Geometry: final body of the model. Coordinates: model frame, mm. Face numbers are marked on the shaded views. Give positions to 0.01 mm unless a question says otherwise; leave off trailing zeros. Order: outer loops, then holes, each group sorted by start corner. A loop starts at its lowest first (then second) coordinate and runs counter-clockwise, first axis right, second up. Notation, with made-up numbers: (3, -6) - (10, -6) arc R25 ccw to (10, 27) - close; hole circle Ø8 at (2, -12.5). An arc over 180 degrees is marked (long way). One line per item, written item: value.
```python
from build123d import *

# Parameters (mm, degrees)
MINUS_PLATE_10_X_8_5_X_0_5_SKETCH_W = 10
MINUS_PLATE_10_X_8_5_X_0_5_SKETCH_H = 0.5
MINUS_PLATE_10_X_8_5_X_0_5_DEPTH    = 8.5
SOLDER_TAB_1_5_X_2_5_SKETCH_W       = 1.5
SOLDER_TAB_1_5_X_2_5_SKETCH_H       = 0.5
SOLDER_TAB_1_5_X_2_5_DEPTH          = 2.5


with BuildPart() as part:
    # Minus Plate 10 x 8.5 x 0.5 Sketch → Minus Plate 10 x 8.5 x 0.5 (new body)
    with BuildSketch(Plane(origin=(0, 1.95, 0), x_dir=(1, 0, 0), z_dir=(0, 1, 0))):
        with Locations((25.7, 65.1)):
            Rectangle(MINUS_PLATE_10_X_8_5_X_0_5_SKETCH_W, MINUS_PLATE_10_X_8_5_X_0_5_SKETCH_H)
    extrude(amount=MINUS_PLATE_10_X_8_5_X_0_5_DEPTH)

    # Solder Tab 1.5 x 2.5 Sketch → Solder Tab 1.5 x 2.5 (add)
    with BuildSketch(Plane(origin=(0, 10.45, 0), x_dir=(1, 0, 0), z_dir=(0, 1, 0))):
        with Locations((25.7, 65.1)):
            Rectangle(SOLDER_TAB_1_5_X_2_5_SKETCH_W, SOLDER_TAB_1_5_X_2_5_SKETCH_H)
    extrude(amount=SOLDER_TAB_1_5_X_2_5_DEPTH)

    # Spring (compressed 4.3) Sketch → Spring (compressed 4.3) (revolve)
    with BuildSketch(Plane(origin=(0, 6.95, 0), x_dir=(1, 0, 0), z_dir=(0, 1, 0)), mode=Mode.PRIVATE) as spring_compressed_4_3_sk:
        Polygon((28.2, 64.85), (28.7, 64.85), (27.7, 60.55), (27.2, 60.55), align=None)
    revolve(spring_compressed_4_3_sk.sketch.rotate(Axis((25.7, 6.95, -65.85), (0, 0, 1)), 180), axis=Axis((25.7, 6.95, -65.85), (0, 0, 1)))


solid = part.part
```
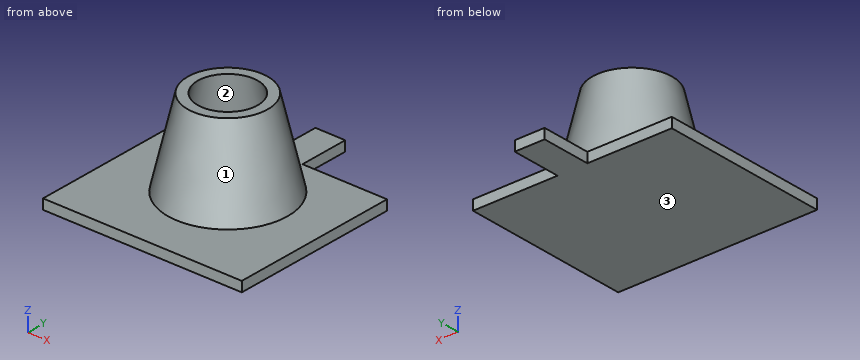
1) Section B-B, the plane y = 6.95. Return loops of the section in (x, z), then the cut area to 3 significant figures.
Answers below:
outline: (20.7, -65.35) - (30.7, -65.35) - (30.7, -64.85) - (28.7, -64.85) - (27.7, -60.55) - (27.2, -60.55) - (28.2, -64.85) - (23.2, -64.85) - (24.2, -60.55) - (23.7, -60.55) - (22.7, -64.85) - (20.7, -64.85) - close
area: 9.30 mm^2
2) Material intervals for line 1 along Y through (x, z) = (26.75, -62.55); line 2 along Y through (x, z) = (24, -62.8); line 3 along Z through (x, y) = (29, 4.5), sorted ascending.
Answers below:
line 1: 4.72 to 5.29, 8.61 to 9.18
line 2: 5.09 to 5.85, 8.05 to 8.81
line 3: -65.35 to -64.85
3) Section D-D, the plane x = 22. Return loops of the section in (y, z).
Answers below:
outline: (1.95, -65.35) - (10.45, -65.35) - (10.45, -64.85) - (1.95, -64.85) - close
4) Section C-C, the plane z = -62.75. Return loops of the section in (x, y), then the cut area to 3 significant figures.
Answers below:
outline: circle Ø5.02 at (25.7, 6.95); hole circle Ø4.02 at (25.7, 6.95)
area: 7.11 mm^2
5) Mould query, pull axis Z, two halves, no side actions, for the marked faces 1, 2 and 3. Classes: released by +Z, released by -Z, zero draft, split by the parting line, or undercut.
Answers below:
face 1: released by +Z
face 2: undercut
face 3: released by -Z
6) Section A-A, the plane x = 25.7. Return loops of the section in (y, z), then the cut area to 3 significant figures.
Answers below:
outline: (1.95, -65.35) - (12.95, -65.35) - (12.95, -64.85) - (9.95, -64.85) - (8.95, -60.55) - (8.45, -60.55) - (9.45, -64.85) - (4.45, -64.85) - (5.45, -60.55) - (4.95, -60.55) - (3.95, -64.85) - (1.95, -64.85) - close
area: 9.80 mm^2
7) First-contact query: pin 1 (1.5 mm diameter, centred on y = 11, z = -63.5, fed in from -X); pin 2 (0.6 mm diameter, centred on x = 22.5, z = -65, fed in from +Y); pin 3 (1.5 mm diameter, centred on x = 26.5, z = -63.5, fed in from +Y); pin 4 (1.5 mm diameter, centred on y = 8, z = -63, fed in from +X). Flat tips, straight axial feed; report the tip coordinate or a pass-through.
Answers below:
pin 1: through
pin 2: y = 10.45
pin 3: y = 9.76
pin 4: x = 28.34
